Geometry: final body of the model. Coordinates: model frame, mm. A direction names the side the tool comes from. Coordinates: 2 decimals unless noted, no trailing zeros. Order: outer loops, then holes, each group sorted by start corner. A loop starts at its lowest first (then second) coordinate and runs counter-clockwise, first axis right, second up. Notation, with made-up numbers: (-12, 83.5) -> (41, 83.5) arc R22 cw to (41, 95.5) -> close; hole circle Ø6 at (85.25, 37.5). An arc over 180 degrees is marked (long way). Answer in a Markdown table with one row per item. Add a question column.
1) Section query A-A on x = 0. Return the cut outline in (y, z).
2) Ray query, line 1 (Y direction, x = -0.5, z = -361.5); line 2 (X direction, y = 1, z = -28.5); line 3 (Z direction, x = -17, y = 143). Return the intervals inside material, ascending. Write a range as from..to.
3) Pull-direction query (Y, two-part tool) for faces 1 (the face through (12.31, 60.88, -65.62)), 2 (the face through (-31.6, 144, -346)); classes: +Y half, -Y half, draft (parallel to the pull), parting line (faces both ways), or undercut.
4) Set-up query: faces 3 (the face through (-0.155, 144.017, -354.368)), 4 (the face through (-23.219, 144.017, -354.368)), 5 (the face through (24.361, 144.017, -354.368)). Return all of +Z, -Z, +X, -X, +Y, -Y with unobstructed straight access to the full face (end or side cutting, diameter ignored); none if empty.
5) Section query B-B on y = 0. Return the cut outline in (x, z).
6) Section query C-C on z = -292. Return the cut outline in (x, y), then the cut area to 3 significant figures.
7) Contact query for flat-ended pins moving along their axis: P1, Ø5, axis at x = 13, z = -214, coming from the -Y side; P2, Ø6, axis at x = 2.5, z = -362, coming from the +Y side; P3, Ø1.5, axis at x = 9, z = -450, coming from the +Y side. Output: stop coordinate, or through.
```python
from build123d import *

# Parameters (mm, degrees)
SKETCH1_R                = 25.8
BOSS_EXTRUDE1_DEPTH      = 544
SKETCH6_R                = 14.6
BOSS_EXTRUDE2_REACH      = 541.822
BOSS_EXTRUDE2_END_RADIUS = 25.8
SKETCH4_R                = 14.6
BOSS_EXTRUDE3_START      = -3.5
BOSS_EXTRUDE3_OUTLINE_R  = 8.35
BOSS_EXTRUDE3_DEPTH      = 3.5
BOSS_EXTRUDE4_START      = 17
SKETCH7_3_R              = 8.35
BOSS_EXTRUDE4_DEPTH      = 66
SKETCH9_R                = 25.8
BOSS_EXTRUDE5_DEPTH      = 16.49
BOSS_EXTRUDE6_START      = 23.51
SKETCH10_R               = 25.8
BOSS_EXTRUDE6_DEPTH      = 23.51
BOSS_EXTRUDE7_START      = 4.5
SKETCH11_R               = 14.6
BOSS_EXTRUDE7_DEPTH      = 4.5


# Read off the part's stored shape, not the designer's step: Boss-Extrude3
with BuildPart() as part:
    # Sketch1 → Boss-Extrude1 (new body)
    with BuildSketch(Plane.XY):
        Circle(SKETCH1_R)
    extrude(amount=-BOSS_EXTRUDE1_DEPTH)

    # Sweep2: sweep along a path in Sketch2
    with BuildLine(Plane(origin=(0, 0, 0), x_dir=(0, 0, -1), z_dir=(1, 0, 0))) as sweep2_path:
        Line((535.242725219, 10.616416132), (373.485286901, 119.6))
        Line((373.485286901, 119.6), (-26.514713099, 119.6))
    # Sketch6 → Sweep2 (sweep)
    with BuildSketch(Plane(origin=(0, 10.616416132, -535.242725219), x_dir=(1, 0, 0), z_dir=(0, 0.5587587437797145, 0.8293302516185669))):
        Circle(SKETCH6_R)
    sweep(path=sweep2_path.line, transition=Transition.RIGHT)

    # Boss-Extrude2: up to this cylinder (the profile starts outside it)
    boss_extrude2_end = Plane(origin=(0, 0, 7.489761), z_dir=(0, 0, 1)) * Cylinder(BOSS_EXTRUDE2_END_RADIUS, 1136.244, mode=Mode.PRIVATE)
    # Sketch4 → Boss-Extrude2 (add, up to the surface)
    with BuildSketch(Plane(origin=(0, 296.142134203, -111.454966642), x_dir=(1, 0, 0), z_dir=(0, 0.5587587437797145, 0.8293302516185669)), mode=Mode.PRIVATE) as boss_extrude2_sk1:
        with Locations(Location((0, -212.87313933, 0), (0, 0, 270))):
            Circle(SKETCH4_R)
    boss_extrude2_tool1 = extrude(boss_extrude2_sk1.sketch, amount=-BOSS_EXTRUDE2_REACH, mode=Mode.PRIVATE) - boss_extrude2_end
    add(boss_extrude2_tool1.solids().sort_by_distance((0, 119.6, 7.489761))[0])

    # Boss-Extrude3 outline → Boss-Extrude3 (add)
    with BuildSketch(Plane.ZY.offset(14.6).offset(BOSS_EXTRUDE3_START)):
        with BuildLine():
            add(Edge.make_bspline(
                [(-369.025798161, 121.314868638), (-354.153662916, 130.263805611), (-368.24558028, 157.483504956), (-346.0257981, 157.599948143)],
                knots=[0, 0, 0, 0, 0.999846057, 0.999846057, 0.999846057, 0.999846057], degree=3))
            Line((-369.025798161, 121.314868638), (-323.025798161, 121.314868638))
            add(Edge.make_bspline(
                [(-323.025798161, 121.314868638), (-337.897933379, 130.263805595), (-323.806016093, 157.483504857), (-346.0257981, 157.599948143)],
                knots=[0, 0, 0, 0, 0.999846056, 0.999846056, 0.999846056, 0.999846056], degree=3))
        make_face()
        with Locations((-346.025798161, 143.65)):
            Circle(BOSS_EXTRUDE3_OUTLINE_R, mode=Mode.SUBTRACT)
    boss_extrude3 = extrude(amount=BOSS_EXTRUDE3_DEPTH)

    # Mirror1: Boss-Extrude3 across plane
    add(boss_extrude3.mirror(Plane.ZY))

    # Sketch7<3> → Boss-Extrude4 (add)
    with BuildSketch(Plane.ZY.offset(14.6).offset(BOSS_EXTRUDE4_START)):
        with Locations((-346.025798161, 143.65)):
            Circle(SKETCH7_3_R)
    extrude(amount=-BOSS_EXTRUDE4_DEPTH)

    # Sketch9 → Boss-Extrude5 (add)
    with BuildSketch(Plane(origin=(0, 0, -544), x_dir=(-1, 0, 0), z_dir=(0, 0, -1))):
        with Locations(Location((0, 0, 0), (0, 0, 180))):
            Circle(SKETCH9_R)
    extrude(amount=BOSS_EXTRUDE5_DEPTH)

    # Sketch10 → Boss-Extrude6 (add)
    with BuildSketch(Plane.XY.offset(BOSS_EXTRUDE6_START)):
        Circle(SKETCH10_R)
    extrude(amount=-BOSS_EXTRUDE6_DEPTH)

    # Sketch11 → Boss-Extrude7 (add)
    with BuildSketch(Plane.XY.offset(26.514713099).offset(BOSS_EXTRUDE7_START)):
        with Locations((0, 119.6)):
            Circle(SKETCH11_R)
    extrude(amount=-BOSS_EXTRUDE7_DEPTH)


solid = part.part
```
Result:
| question | item | result |
|---|---|---|
| 1 | outline | (-25.8, -560.49) -> (25.8, -560.49) -> (25.8, -538.84) -> (134.2, -377.94) -> (134.2, 31.01) -> (105, 31.01) -> (105, 11.95) -> (25.8, -105.6) -> (25.8, 23.51) -> (-25.8, 23.51) -> close; circle Ø16.7 at (143.65, -346.03); hole (25.8, -486.58) -> (105, -369.03) -> (105, -40.31) -> (25.8, -157.86) -> close |
| 2 | line 1 | -25.8..25.8, 105.01..134.19 |
| 2 | line 2 | -25.78..25.78 |
| 2 | line 3 | -354.35..-337.7 |
| 3 | face 1 | undercut |
| 3 | face 2 | draft |
| 4 | face 3 | none |
| 4 | face 4 | -X |
| 4 | face 5 | +X |
| 5 | outline | (-25.8, -560.49) -> (25.8, -560.49) -> (25.8, 23.51) -> (-25.8, 23.51) -> close |
| 6 | outline | circle Ø51.6 at (0, 0); circle Ø29.2 at (0, 119.6) |
| 6 | area | 2,760 mm2 |
| 7 | P1 | y = -23.57 |
| 7 | P2 | y = 134.2 |
| 7 | P3 | y = 82.75 |
